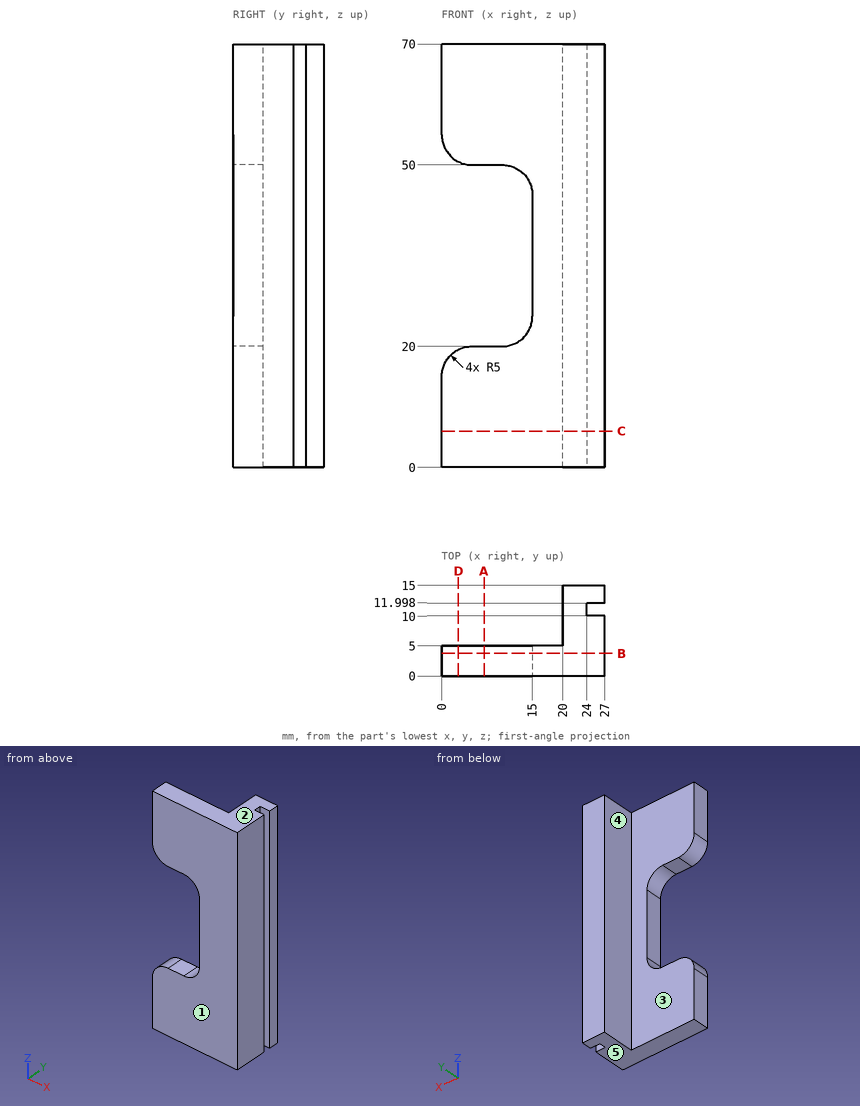
For this review, use the dimensioned drawing (mm, ordinates from the lowest corner) and the shaded views. A direction names the side the tool comes from. Give positions to 0.01 mm unless a question says otherwise; leave off trailing zeros. Loops run counter-clockwise (first coordinate to the right, second up) from the corner with the lowest first, then second, coordinate; pieces in that order, holes last.
Item 1: Take a section at C-C, the plane z = 6. State the section outline as (x, y) points, and give its area (3 significant figures).
Item 2: Insertion check: pin 1 (12 mm diameter, centred on x = 6, z = 33.5, fed in from +Y); pin 2 (8 mm diameter, centred on y = 10, z = 44, fed in from -X); pin 3 (5.5 mm diameter, centred on y = 3.5, z = 39, fed in from -X); pin 4 (10 mm diameter, centred on x = 12.5, z = 47.5, fed in from +Y). Each pin has a flat end and moves straight along its axis. Give the tip position at first contact, or say it passes through.
Item 3: For line 1 along Y through (x, z) = (26, 23.5); line 2 along Z through (x, y) = (6.25, 1.5); line 3 along Y through (x, z) = (1.25, 17), list the stretches that pass through material, from the lowest coordinate up.
Item 4: Take a section at A-A, the plane x = 7. State the section outline as (y, z) points.
Item 5: Draft analysis for pull direction Y (two halves, no side actions). For the marked faces 1, 2 and 3, state which applies: +Y half, -Y half, draft (parallel to the pull), parting line (faces both ways), or undercut.
Item 6: Tool access review of the marked faces 4 and 5: name each direction out of +Z, -Z, +X, -X, +Y, -Y from which nothing blocks a thin tool from reaching the whole face with its end or side.
Item 7: Take a section at B-B, the plane y = 3.75. State the section outline as (x, z) points, and give its area (3 significant figures).
Item 8: Take a section at D-D, the plane x = 2.75. State the section outline as (y, z) points (3 decimals), and give its area (3 significant figures).
Calculated:
1. outline: (0, 0) - (27, 0) - (27, 10) - (24, 10) - (24, 12) - (27, 12) - (27, 15) - (20, 15) - (20, 5) - (0, 5) - close
1. area: 199 mm2
2. pin 1: passes through
2. pin 2: stops at x = 20
2. pin 3: stops at x = 15
2. pin 4: stops at y = 5
3. line 1: y = 0 to 10, 12 to 15
3. line 2: z = 0 to 20, 50 to 70
3. line 3: y = 0 to 5
4. outline: (0, 0) - (5, 0) - (5, 20) - (0, 20) - close; (0, 50) - (5, 50) - (5, 70) - (0, 70) - close
5. face 1: -Y half
5. face 2: draft
5. face 3: +Y half
6. face 4: +Z, -Z, -X, +Y
6. face 5: -Z, +X, -X, +Y, -Y
7. outline: (0, 0) - (27, 0) - (27, 70) - (0, 70) - (0, 55) arc R5 ccw to (5, 50) - (10, 50) arc R5 cw to (15, 45) - (15, 25) arc R5 cw to (10, 20) - (5, 20) arc R5 ccw to (0, 15) - close
7. area: 1,440 mm2
8. outline: (0, 0) - (5, 0) - (5, 19.465) - (0, 19.465) - close; (0, 50.535) - (5, 50.535) - (5, 70) - (0, 70) - close
8. area: 195 mm2
